from build123d import *

# Parameters (mm, degrees)
F0_R     = 76.2
F1_DEPTH = 25.4
F3_R     = 16.891
F4_DEPTH = 25.4


with BuildPart() as f1:
    # F0 (on Front) → F1 (new body)
    with BuildSketch(Plane.XZ):
        Circle(F0_R)
    extrude(amount=F1_DEPTH)

    # F3 (on face) → F4 (cut)
    with BuildSketch(Plane.XZ.offset(25.4)):
        with Locations((35.921024, 35.921024)):
            Circle(F3_R)
        with BuildLine():
            ThreePointArc((21.266493, -26.411296), (11.274742, -31.979688), (0, -33.909))
            ThreePointArc((0, -33.909), (-16.891, -50.8), (0, -67.691))
            ThreePointArc((0, -67.691), (22.507258, -63.839602), (42.453336, -52.723674))
            ThreePointArc((42.453336, -52.723674), (45.016103, -28.974064), (21.266493, -26.411296))
        make_face()
        with Locations((-50.506798, 5.450076)):
            Circle(F3_R)
    extrude(amount=-F4_DEPTH, mode=Mode.SUBTRACT)


solid = f1.part
Input: part model. Units: mm. Frame: model coordinates. A direction names the side the tool comes from. Coordinates: 2 decimals unless noted, no trailing zeros. Write each loop counter-clockwise with the first axis right and the second up, starting at its lowest first coordinate (ties: lowest second). Pieces come first, ordered by that corner, then holes. Notation, with made-up numbers: M 40.25,-7.5 L 63.25,-7.5 A19 cw 63.25,7.5 Z; hole C 28.25,23.5 d10. An arc over 180 degrees is marked long. Answer as a JSON object with one key per item and string values. Group by question number.
(1) Section B-B on x = 35.5. Output: boundary loops of the cut face in (y, z).
(2) Section D-D on y = -21.5. Output: boundary loops of the cut face in (x, z).
(3) Section C-C on x = 12.5. Output: boundary loops of the cut face in (y, z).
(4) Contact query for flat-ended pins moving along their axis: P1, Ø1.5, axis at x = -40, y = -3, coming from the -Z side; P2, Ø1, axis at x = 34.5, y = -4, coming from the -Z side; P3, Ø6, axis at y = -21, z = 37.5, coming from the +X side. Output: stop coordinate, or through.
(5) Set-up query: faces 1 (the face through (22.204, -12.878, -63.946)), 2 (the face through (-1, -25.4, 1)). Return all of +Z, -Z, +X, -X, +Y, -Y with unobstructed straight access to the full face (end or side cutting, diameter ignored); none if empty.
(6) Section A-A on z = -5.5. Output: boundary loops of the cut face in (x, y), plus the area to 3 significant figures.
(7) Ray query, line 1 along Z through (x, y) = (43.5, -1.75); line 2 along X through (y, z) = (-9, -27); line 3 along X through (y, z) = (-21, 16.5). Return the intervals inside material, ascending. Write a range as [from, to].
(8) Mould query, pull axis X, two halves, no side actions, for faces 3 (the face through (-1, 0, 1)), 4 (the face through (22.52, -12.88, 25.64)), 5 (the face through (-60.47, -12.522, -46.367)). Classes: pulls with the +X half, pulls with the -X half, needs draft (parallel to the pull), parting line crosses it, or undercut.
Result set:
{
 "1": {"outline": "M -25.4,-67.43 L 0,-67.43 L 0,-57.64 L -25.4,-57.64 Z; M -25.4,-23.07 L 0,-23.07 L 0,19.04 L -25.4,19.04 Z; M -25.4,52.81 L 0,52.81 L 0,67.43 L -25.4,67.43 Z"},
 "2": {"outline": "C 0,0 d152.4; hole C -50.51,5.45 d33.78; hole M 0,-67.69 A67.69 ccw 42.45,-52.72 A16.89 ccw 21.27,-26.41 A33.91 cw 0,-33.91 A16.89 ccw Z; hole C 35.92,35.92 d33.78"},
 "3": {"outline": "M -25.4,-75.17 L 0,-75.17 L 0,-66.53 L -25.4,-66.53 Z; M -25.4,-31.52 L 0,-31.52 L 0,75.17 L -25.4,75.17 Z"},
 "4": {"P1": "stops at z = -65.31", "P2": "stops at z = -68.19", "P3": "stops at x = 67.94"},
 "5": {"face 1": "+Y, -Y", "face 2": "+Z, -Z, +X, -X, -Y"},
 "6": {"outline": "M -76,-25.4 L -63.37,-25.4 L -63.37,0 L -76,0 Z; M -37.65,-25.4 L 76,-25.4 L 76,0 L -37.65,0 Z", "area": "3,210 mm2"},
 "7": {"line 1": "z = [-62.56, -51.81], [-27.33, 20.83], [51.02, 62.56]", "line 2": "x = [-71.26, 20.51], [43.15, 71.26]", "line 3": "x = [-74.39, -63.28], [-37.73, 74.39]"},
 "8": {"face 3": "needs draft", "face 4": "undercut", "face 5": "parting line crosses it"}
}
